Input: part model. Units: mm. Frame: model coordinates. A direction names the side the tool comes from. Round coordinates to 2 decimals unless told otherwise and drop trailing zeros. Order: outer loops, then holes, each group sorted by start corner. A loop starts at its lowest first (then second) coordinate and runs counter-clockwise, first axis right, second up. Notation, with made-up numbers: (88.25, -17) - (131.25, -17) arc R11 ccw to (131.25, 3) - close; hole circle Ø3 at (3, -14). An arc over 180 degrees is marked (long way). One line per item, written item: value. Start each with the question number.
from build123d import *

# Parameters (mm, degrees)
EXTRUDE_THIN1_OUTLINE_W      = 19.7612
EXTRUDE_THIN1_OUTLINE_H      = 19.7612
EXTRUDE_THIN1_OUTLINE_W_2    = 18.2372
EXTRUDE_THIN1_OUTLINE_H_2    = 18.2372
EXTRUDE_THIN1_DEPTH          = 6.52585
EXTRUDE_THIN1_2_OUTLINE_W    = 15.748
EXTRUDE_THIN1_2_OUTLINE_H    = 9.652
EXTRUDE_THIN1_2_OUTLINE_W_2  = 14.224
EXTRUDE_THIN1_2_OUTLINE_H_2  = 8.128
EXTRUDE_THIN1_2_DEPTH        = 6.52585
EXTRUDE_THIN1_3_OUTLINE_W    = 15.748
EXTRUDE_THIN1_3_OUTLINE_H    = 9.652
EXTRUDE_THIN1_3_OUTLINE_W_2  = 14.224
EXTRUDE_THIN1_3_OUTLINE_H_2  = 8.128
EXTRUDE_THIN1_3_DEPTH        = 6.52585
EXTRUDE_THIN1_4_OUTLINE_W    = 15.748
EXTRUDE_THIN1_4_OUTLINE_H    = 9.652
EXTRUDE_THIN1_4_OUTLINE_W_2  = 14.224
EXTRUDE_THIN1_4_OUTLINE_H_2  = 8.128
EXTRUDE_THIN1_4_DEPTH        = 6.52585
EXTRUDE_THIN1_5_OUTLINE_W    = 15.748
EXTRUDE_THIN1_5_OUTLINE_H    = 9.652
EXTRUDE_THIN1_5_OUTLINE_W_2  = 14.224
EXTRUDE_THIN1_5_OUTLINE_H_2  = 8.128
EXTRUDE_THIN1_5_DEPTH        = 6.52585
EXTRUDE_THIN1_6_OUTLINE_W    = 15.748
EXTRUDE_THIN1_6_OUTLINE_H    = 9.652
EXTRUDE_THIN1_6_OUTLINE_W_2  = 14.224
EXTRUDE_THIN1_6_OUTLINE_H_2  = 8.128
EXTRUDE_THIN1_6_DEPTH        = 6.52585
EXTRUDE_THIN1_7_OUTLINE_W    = 15.748
EXTRUDE_THIN1_7_OUTLINE_H    = 9.652
EXTRUDE_THIN1_7_OUTLINE_W_2  = 14.224
EXTRUDE_THIN1_7_OUTLINE_H_2  = 8.128
EXTRUDE_THIN1_7_DEPTH        = 6.52585
EXTRUDE_THIN1_8_OUTLINE_W    = 15.748
EXTRUDE_THIN1_8_OUTLINE_H    = 9.652
EXTRUDE_THIN1_8_OUTLINE_W_2  = 14.224
EXTRUDE_THIN1_8_OUTLINE_H_2  = 8.128
EXTRUDE_THIN1_8_DEPTH        = 6.52585
EXTRUDE_THIN1_9_OUTLINE_W    = 15.748
EXTRUDE_THIN1_9_OUTLINE_H    = 9.652
EXTRUDE_THIN1_9_OUTLINE_W_2  = 14.224
EXTRUDE_THIN1_9_OUTLINE_H_2  = 8.128
EXTRUDE_THIN1_9_DEPTH        = 6.52585
EXTRUDE_THIN1_10_OUTLINE_W   = 15.748
EXTRUDE_THIN1_10_OUTLINE_H   = 9.652
EXTRUDE_THIN1_10_OUTLINE_W_2 = 14.224
EXTRUDE_THIN1_10_OUTLINE_H_2 = 8.128
EXTRUDE_THIN1_10_DEPTH       = 6.52585
EXTRUDE_THIN1_11_OUTLINE_W   = 15.748
EXTRUDE_THIN1_11_OUTLINE_H   = 9.652
EXTRUDE_THIN1_11_OUTLINE_W_2 = 14.224
EXTRUDE_THIN1_11_OUTLINE_H_2 = 8.128
EXTRUDE_THIN1_11_DEPTH       = 6.52585
EXTRUDE_THIN1_12_OUTLINE_W   = 15.748
EXTRUDE_THIN1_12_OUTLINE_H   = 9.652
EXTRUDE_THIN1_12_OUTLINE_W_2 = 14.224
EXTRUDE_THIN1_12_OUTLINE_H_2 = 8.128
EXTRUDE_THIN1_12_DEPTH       = 6.52585
EXTRUDE_THIN1_13_OUTLINE_W   = 19.7612
EXTRUDE_THIN1_13_OUTLINE_H   = 19.7612
EXTRUDE_THIN1_13_OUTLINE_W_2 = 18.2372
EXTRUDE_THIN1_13_OUTLINE_H_2 = 18.2372
EXTRUDE_THIN1_13_DEPTH       = 6.52585
BOSS_EXTRUDE1_START          = -6.52585
SKETCH3_W                    = 1.397
SKETCH3_H                    = 45.6184
SKETCH3_W_2                  = 3.2004
SKETCH3_H_2                  = 19.7612
SKETCH3_W_3                  = 4.212549516
BOSS_EXTRUDE1_DEPTH          = 6.52585
FILLET1_R                    = 3.302


# Read off the part's stored shape, not the designer's step: Extrude-Thin1
with BuildPart() as part:
    # Extrude-Thin1 outline → Extrude-Thin1 (new body)
    with BuildSketch(Plane.XY):
        with Locations((610.948497092, 512.7244)):
            Rectangle(EXTRUDE_THIN1_OUTLINE_W, EXTRUDE_THIN1_OUTLINE_H)
        with Locations((610.948497092, 512.7244)):
            Rectangle(EXTRUDE_THIN1_OUTLINE_W_2, EXTRUDE_THIN1_OUTLINE_H_2, mode=Mode.SUBTRACT)
    extrude(amount=EXTRUDE_THIN1_DEPTH)



with BuildPart() as body_2:
    # Extrude-Thin1 2 outline → Extrude-Thin1 2 (new body)
    with BuildSketch(Plane.XY):
        with Locations((548.874747576, 544.195)):
            Rectangle(EXTRUDE_THIN1_2_OUTLINE_W, EXTRUDE_THIN1_2_OUTLINE_H)
        with Locations((548.874747576, 544.195)):
            Rectangle(EXTRUDE_THIN1_2_OUTLINE_W_2, EXTRUDE_THIN1_2_OUTLINE_H_2, mode=Mode.SUBTRACT)
    extrude(amount=EXTRUDE_THIN1_2_DEPTH)


with BuildPart() as body_3:
    # Extrude-Thin1 3 outline → Extrude-Thin1 3 (new body)
    with BuildSketch(Plane.XY):
        with Locations((548.874747576, 535.2034)):
            Rectangle(EXTRUDE_THIN1_3_OUTLINE_W, EXTRUDE_THIN1_3_OUTLINE_H)
        with Locations((548.874747576, 535.2034)):
            Rectangle(EXTRUDE_THIN1_3_OUTLINE_W_2, EXTRUDE_THIN1_3_OUTLINE_H_2, mode=Mode.SUBTRACT)
    extrude(amount=EXTRUDE_THIN1_3_DEPTH)


with BuildPart() as body_4:
    # Extrude-Thin1 4 outline → Extrude-Thin1 4 (new body)
    with BuildSketch(Plane.XY):
        with Locations((548.874747576, 526.2118)):
            Rectangle(EXTRUDE_THIN1_4_OUTLINE_W, EXTRUDE_THIN1_4_OUTLINE_H)
        with Locations((548.874747576, 526.2118)):
            Rectangle(EXTRUDE_THIN1_4_OUTLINE_W_2, EXTRUDE_THIN1_4_OUTLINE_H_2, mode=Mode.SUBTRACT)
    extrude(amount=EXTRUDE_THIN1_4_DEPTH)


with BuildPart() as body_5:
    # Extrude-Thin1 5 outline → Extrude-Thin1 5 (new body)
    with BuildSketch(Plane.XY):
        with Locations((548.874747576, 517.2202)):
            Rectangle(EXTRUDE_THIN1_5_OUTLINE_W, EXTRUDE_THIN1_5_OUTLINE_H)
        with Locations((548.874747576, 517.2202)):
            Rectangle(EXTRUDE_THIN1_5_OUTLINE_W_2, EXTRUDE_THIN1_5_OUTLINE_H_2, mode=Mode.SUBTRACT)
    extrude(amount=EXTRUDE_THIN1_5_DEPTH)


with BuildPart() as body_6:
    # Extrude-Thin1 6 outline → Extrude-Thin1 6 (new body)
    with BuildSketch(Plane.XY):
        with Locations((548.874747576, 508.2286)):
            Rectangle(EXTRUDE_THIN1_6_OUTLINE_W, EXTRUDE_THIN1_6_OUTLINE_H)
        with Locations((548.874747576, 508.2286)):
            Rectangle(EXTRUDE_THIN1_6_OUTLINE_W_2, EXTRUDE_THIN1_6_OUTLINE_H_2, mode=Mode.SUBTRACT)
    extrude(amount=EXTRUDE_THIN1_6_DEPTH)


with BuildPart() as body_7:
    # Extrude-Thin1 7 outline → Extrude-Thin1 7 (new body)
    with BuildSketch(Plane.XY):
        with Locations((548.874747576, 499.237)):
            Rectangle(EXTRUDE_THIN1_7_OUTLINE_W, EXTRUDE_THIN1_7_OUTLINE_H)
        with Locations((548.874747576, 499.237)):
            Rectangle(EXTRUDE_THIN1_7_OUTLINE_W_2, EXTRUDE_THIN1_7_OUTLINE_H_2, mode=Mode.SUBTRACT)
    extrude(amount=EXTRUDE_THIN1_7_DEPTH)


with BuildPart() as body_8:
    # Extrude-Thin1 8 outline → Extrude-Thin1 8 (new body)
    with BuildSketch(Plane.XY):
        with Locations((566.019747576, 499.237)):
            Rectangle(EXTRUDE_THIN1_8_OUTLINE_W, EXTRUDE_THIN1_8_OUTLINE_H)
        with Locations((566.019747576, 499.237)):
            Rectangle(EXTRUDE_THIN1_8_OUTLINE_W_2, EXTRUDE_THIN1_8_OUTLINE_H_2, mode=Mode.SUBTRACT)
    extrude(amount=EXTRUDE_THIN1_8_DEPTH)


with BuildPart() as body_9:
    # Extrude-Thin1 9 outline → Extrude-Thin1 9 (new body)
    with BuildSketch(Plane.XY):
        with Locations((566.019747576, 508.2286)):
            Rectangle(EXTRUDE_THIN1_9_OUTLINE_W, EXTRUDE_THIN1_9_OUTLINE_H)
        with Locations((566.019747576, 508.2286)):
            Rectangle(EXTRUDE_THIN1_9_OUTLINE_W_2, EXTRUDE_THIN1_9_OUTLINE_H_2, mode=Mode.SUBTRACT)
    extrude(amount=EXTRUDE_THIN1_9_DEPTH)


with BuildPart() as body_10:
    # Extrude-Thin1 10 outline → Extrude-Thin1 10 (new body)
    with BuildSketch(Plane.XY):
        with Locations((566.019747576, 517.2202)):
            Rectangle(EXTRUDE_THIN1_10_OUTLINE_W, EXTRUDE_THIN1_10_OUTLINE_H)
        with Locations((566.019747576, 517.2202)):
            Rectangle(EXTRUDE_THIN1_10_OUTLINE_W_2, EXTRUDE_THIN1_10_OUTLINE_H_2, mode=Mode.SUBTRACT)
    extrude(amount=EXTRUDE_THIN1_10_DEPTH)


with BuildPart() as body_11:
    # Extrude-Thin1 11 outline → Extrude-Thin1 11 (new body)
    with BuildSketch(Plane.XY):
        with Locations((566.019747576, 535.2034)):
            Rectangle(EXTRUDE_THIN1_11_OUTLINE_W, EXTRUDE_THIN1_11_OUTLINE_H)
        with Locations((566.019747576, 535.2034)):
            Rectangle(EXTRUDE_THIN1_11_OUTLINE_W_2, EXTRUDE_THIN1_11_OUTLINE_H_2, mode=Mode.SUBTRACT)
    extrude(amount=EXTRUDE_THIN1_11_DEPTH)


with BuildPart() as body_12:
    # Extrude-Thin1 12 outline → Extrude-Thin1 12 (new body)
    with BuildSketch(Plane.XY):
        with Locations((566.019747576, 526.2118)):
            Rectangle(EXTRUDE_THIN1_12_OUTLINE_W, EXTRUDE_THIN1_12_OUTLINE_H)
        with Locations((566.019747576, 526.2118)):
            Rectangle(EXTRUDE_THIN1_12_OUTLINE_W_2, EXTRUDE_THIN1_12_OUTLINE_H_2, mode=Mode.SUBTRACT)
    extrude(amount=EXTRUDE_THIN1_12_DEPTH)


with BuildPart() as body_13:
    # Extrude-Thin1 13 outline → Extrude-Thin1 13 (new body)
    with BuildSketch(Plane.XY):
        with Locations((586.974747576, 512.7244)):
            Rectangle(EXTRUDE_THIN1_13_OUTLINE_W, EXTRUDE_THIN1_13_OUTLINE_H)
        with Locations((586.974747576, 512.7244)):
            Rectangle(EXTRUDE_THIN1_13_OUTLINE_W_2, EXTRUDE_THIN1_13_OUTLINE_H_2, mode=Mode.SUBTRACT)
    extrude(amount=EXTRUDE_THIN1_13_DEPTH)


with BuildPart() as part_1:
    add(part.part)

    add(body_2.part)  # Boss-Extrude1 merges body 2

    add(body_3.part)  # Boss-Extrude1 merges body 3

    add(body_4.part)  # Boss-Extrude1 merges body 4

    add(body_5.part)  # Boss-Extrude1 merges body 5

    add(body_6.part)  # Boss-Extrude1 merges body 6

    add(body_7.part)  # Boss-Extrude1 merges body 7

    add(body_8.part)  # Boss-Extrude1 merges body 8

    add(body_9.part)  # Boss-Extrude1 merges body 9

    add(body_10.part)  # Boss-Extrude1 merges body 10

    add(body_11.part)  # Boss-Extrude1 merges body 11

    add(body_12.part)  # Boss-Extrude1 merges body 12

    add(body_13.part)  # Boss-Extrude1 merges body 13
    # Sketch3 → Boss-Extrude1 (add)
    with BuildSketch(Plane.XY.offset(6.52585).offset(BOSS_EXTRUDE1_START)):
        with Locations((557.447247576, 517.2202)):
            Rectangle(SKETCH3_W, SKETCH3_H)
        with Locations((575.493947576, 512.7244)):
            Rectangle(SKETCH3_W_2, SKETCH3_H_2)
        with Locations((598.961622334, 512.7244)):
            Rectangle(SKETCH3_W_3, SKETCH3_H_2)
    extrude(amount=BOSS_EXTRUDE1_DEPTH)

    # Fillet1
    fillet1_edges = [part_1.edges().sort_by_distance(p)[0] for p in [
        (556.748747576, 540.0294, 3.262925),
        (573.893747576, 502.8438, 3.262925),
        (573.893747576, 522.605, 3.262925),
    ]]
    fillet(fillet1_edges, radius=FILLET1_R)


solid = part_1.part
Item 1: First-contact query: pin 1 Ø2 at (y, z) = (500, 2) entering from +X; pin 2 Ø3 at (x, z) = (608, 3.5) entering from +Y (3 decimals); pin 3 Ø3 at (x, z) = (595.5, 1) entering from -Y; pin 4 Ø2 at (x, y) = (564.5, 501) entering from -Z. Flat tips, straight axial feed; report the tip coordinate or a pass-through.
Item 2: Section query B-B on y = 506. Return loops of the section in (x, z).
Item 3: Section query C-C on y = 529. Return loops of the section in (x, z).
Item 4: Section query D-D on x = 603. Return loops of the section in (y, z) (3 decimals).
Item 5: Reachability of faces 5 (the face through (549, 549.021, 3)), 6 (the face through (556.749, 546, 3)), 7 (the face through (599, 502.844, 3)), 8 (the face through (555.987, 544, 3)) from +Z, -Z, +X, -X, +Y, -Y: full face, straight path, thin tool, end or side. Return the list, or none.
Item 6: Pull-direction query (Y, two-part tool) for faces 1 (the face through (566, 539.267, 3)), 2 (the face through (566, 531.139, 3)), 3 (the face through (620.829, 513, 3)), 4 (the face through (557, 494.411, 3)); classes: released by +Y, released by -Y, zero draft, split by the parting line, or undercut.
Item 7: Line query: L1, parallel to X at y = 534.5, z = 3.75; L2, parallel to Y at x = 573, z = 0.5; L3, parallel to X at y = 520, z = 1.75. Output: solid intervals per line, ascending.
Item 8: Section query A-A on x = 553.5. Return loops of the section in (y, z), and give its area (3 significant figures).
Geometry results:
1. pin 1: stops at x = 574.23
1. pin 2: stops at y = 522.605
1. pin 3: stops at y = 502.84
1. pin 4: passes through
2. outline: (541, 0) - (541.76, 0) - (541.76, 6.53) - (541, 6.53) - close; (555.99, 0) - (558.91, 0) - (558.91, 6.53) - (555.99, 6.53) - close; (573.13, 0) - (577.86, 0) - (577.86, 6.53) - (573.13, 6.53) - close; (596.09, 0) - (601.83, 0) - (601.83, 6.53) - (596.09, 6.53) - close; (620.07, 0) - (620.83, 0) - (620.83, 6.53) - (620.07, 6.53) - close
3. outline: (541, 0) - (541.76, 0) - (541.76, 6.53) - (541, 6.53) - close; (555.99, 0) - (558.91, 0) - (558.91, 6.53) - (555.99, 6.53) - close; (573.13, 0) - (573.89, 0) - (573.89, 6.53) - (573.13, 6.53) - close
4. outline: (502.844, 0) - (503.606, 0) - (503.606, 6.526) - (502.844, 6.526) - close; (521.843, 0) - (522.605, 0) - (522.605, 6.526) - (521.843, 6.526) - close
5. face 5: +Z, -Z, +X, -X, +Y
5. face 6: +Z, -Z, +X, +Y
5. face 7: +Z, -Z, +X, -Y
5. face 8: +Z, -Z
6. face 1: undercut
6. face 2: undercut
6. face 3: zero draft
6. face 4: released by -Y
7. L1: x = 541 to 541.76, 555.99 to 558.91, 573.13 to 573.89
7. L2: y = 494.41 to 495.17, 503.3 to 504.16, 512.29 to 513.16, 521.28 to 522.15, 530.28 to 531.14, 539.27 to 540.03
7. L3: x = 541 to 541.76, 555.99 to 558.91, 573.13 to 577.86, 596.09 to 601.83, 620.07 to 620.83
8. outline: (494.41, 0) - (495.17, 0) - (495.17, 6.53) - (494.41, 6.53) - close; (503.3, 0) - (504.16, 0) - (504.16, 6.53) - (503.3, 6.53) - close; (512.29, 0) - (513.16, 0) - (513.16, 6.53) - (512.29, 6.53) - close; (521.28, 0) - (522.15, 0) - (522.15, 6.53) - (521.28, 6.53) - close; (530.28, 0) - (531.14, 0) - (531.14, 6.53) - (530.28, 6.53) - close; (539.27, 0) - (540.13, 0) - (540.13, 6.53) - (539.27, 6.53) - close; (548.26, 0) - (549.02, 0) - (549.02, 6.53) - (548.26, 6.53) - close
8. area: 38.1 mm^2
